Read the model definition and answer for the solid it produces. Units are mm, in the model's axes. A direction names the side the tool comes from. Round coordinates to 2 decimals unless told otherwise and drop trailing zeros. Order: outer loops, then holes, each group sorted by start corner. A loop starts at its lowest first (then second) coordinate and runs counter-clockwise, first axis right, second up. Notation, with made-up numbers: (29.5, 32) -> (39.5, 32) arc R15 ccw to (39.5, 60) -> close; hole circle Ø3 at (-9, -24.75). An arc over 180 degrees is marked (long way). Answer as a JSON object with one key per item and string values. Group by question number.
Item 1: Consider probe 1 along Y at (x, z) = (30, 6.25); probe 2 along Z at (x, y) = (-19, -1); probe 3 along X at (y, z) = (4.75, 8.5). Determine where each line is inside the solid, lowest interval first. Write a range as from..to.
Item 2: For faces 5 (the flat face through (-1, 0, 0)), 6 (the flat face through (48, 0, 9)), determine the directions among +Z, -Z, +X, -X, +Y, -Y from which every point of the face is accessible in a straight line to the end or side of a thin tool.
Item 3: The mould has two halves that part along Y. Classify faces 1 (the flat face through (-1, 0, 19)), 2 (the flat face through (-1, -10, 9)), 3 (the flat face through (-1, 0, 2)), 4 (the flat face through (-1, 10, 9)): pulls with the +Y half, pulls with the -Y half, needs draft (parallel to the pull), parting line crosses it, or undercut.
Item 4: Section B-B, the plane y = -5.5 is taken. Write down the section's boundary in (x, z), plus the area to 3 significant figures.
Item 5: Section A-A, the plane z = 3 is taken. Write down the section's boundary in (x, y), plus the area to 3 significant figures.
from build123d import *

# Parameters (mm, degrees)
SKETCH_1_W      = 100
SKETCH_1_H      = 20
EXTRUDE_1_DEPTH = 19
SKETCH_1_2_W    = 100
SKETCH_1_2_H    = 20
EXTRUDE_2_DEPTH = 19
SHELL_1_T       = -2
SKETCH_2_W      = 15
SKETCH_2_H      = 16
EXTRUDE_3_DEPTH = 2


with BuildPart() as part:
    # 草圖1 → 填料-伸長1 (new body)
    with BuildSketch(Plane.XY):
        Rectangle(SKETCH_1_W, SKETCH_1_H)
    extrude(amount=EXTRUDE_1_DEPTH)

    # 草圖1<2> → 填料-伸長2 (add)
    with BuildSketch(Plane.XY):
        Rectangle(SKETCH_1_2_W, SKETCH_1_2_H)
    extrude(amount=EXTRUDE_2_DEPTH)

    # 薄殼1
    shell_1_openings = [part.faces().sort_by_distance(p)[0] for p in [
        (-50, 0, 9.5),
    ]]
    offset(amount=SHELL_1_T, openings=shell_1_openings, kind=Kind.INTERSECTION)

    # 草圖2 → 填料-伸長3 (add)
    with BuildSketch(Plane.ZY.offset(50)):
        with Locations((9.5, 0)):
            Rectangle(SKETCH_2_W, SKETCH_2_H)
    extrude(amount=-EXTRUDE_3_DEPTH)


solid = part.part
Values found:
{
 "1": {"probe 1": "-10..-8, 8..10", "probe 2": "0..2, 17..19", "probe 3": "-50..-48, 48..50"},
 "2": {"face 5": "-Z, +X, -X, +Y, -Y", "face 6": "none"},
 "3": {"face 1": "needs draft", "face 2": "pulls with the -Y half", "face 3": "undercut", "face 4": "pulls with the +Y half"},
 "4": {"outline": "(-50, 0) -> (50, 0) -> (50, 19) -> (-50, 19) -> close; hole (-48, 2) -> (48, 2) -> (48, 17) -> (-48, 17) -> close", "area": "460 mm2"},
 "5": {"outline": "(-50, -10) -> (50, -10) -> (50, 10) -> (-50, 10) -> close; hole (-48, -8) -> (48, -8) -> (48, 8) -> (-48, 8) -> close", "area": "464 mm2"}
}
